Part model, mm, in its own coordinate system. A direction names the side the tool comes from. Round coordinates to 2 decimals unless told otherwise and drop trailing zeros. Loops run counter-clockwise (first coordinate to the right, second up) from the corner with the lowest first, then second, coordinate; pieces in that order, holes last. Notation, with made-up numbers: M 71,23.5 L 87,23.5 A20 cw 87,45.5 Z; hole C -13,70 d8. An arc over 180 degrees is marked long. Put each result on its own line as item: value. Start each with the question number.
1) Drop flat-ended pins along their axis: pin 1 Ø2 at (x, y) = (-1.5, -26.5) entering from -Z; pin 2 Ø1 at (x, y) = (2.5, -25) entering from -Z; pin 3 Ø0.7 at (x, z) = (-2.5, -2) entering from +Y; pin 4 Ø1.5 at (x, z) = (-1.5, -1) entering from -Y. Give the stop position or say it passes through.
2) Pull direction X, two halves, no side cores. Call faces 1 (the flat face through (-3, -36.5, -3)), 2 (the flat face through (2.8, 0, 1.9)): +X half, -X half, draft (parallel to the pull), parting line (faces both ways), or undercut.
3) Slice it at B-B on z = 0. Give the cut face in (x, y), then the cut area to 3 significant figures.
4) Which spindle directions (+Z, -Z, +X, -X, +Y, -Y) get a long thin tool onto all of the face, cutting with end or side? Do faces 3 (the flat face through (-2.7, -13.9, -2.15)), 4 (the flat face through (3.75, -14, 0)), 5 (the cylindrical face through (-3.8, -29.16, 2.11)), 6 (the flat face through (2.8, -27.5, 1.9)). Say none if no direction does.
5) Slice it at A-A on x = 0. Give the cut face in (y, z), then the cut area to 3 significant figures.
6) Probe line 1 along X through (y, z) = (0.5, 0.25); line 2 along Z through (x, y) = (0, -29.75); line 3 along Z through (x, y) = (2.75, -3.5). List the from-to ranges inside material, lowest first.
7) Slice it at C-C on y = -34.75. Give the cut face in (x, z), then the cut area to 3 significant figures.
```python
from build123d import *

# Parameters (mm, degrees)
F3_R      = 4.5
F4_DEPTH  = 27.5
F8_DEPTH  = 27.5
F6_R      = 4.5
F6_R_2    = 4
F9_DEPTH  = 9
F7_R      = 4.5
F7_R_2    = 4
F10_DEPTH = 11
F11_R     = 2.5
F11_R_2   = 0.75
F12_DEPTH = 4.501


# Not quite as in the source:
# - ends of sketch curves that miss each other by under 0.0002 mm in the source are joined


with BuildPart() as f4:
    # F3 (on Front) → F4 (new body)
    with BuildSketch(Plane.XZ):
        Circle(F3_R)
    extrude(amount=F4_DEPTH)

    # F5 (on face) → F8 (cut, through all)
    with BuildSketch(Plane.XZ.offset(27.5)):
        with BuildLine():
            Line((-1.25, -3.8), (0, -3.8))
            Line((0, -3.8), (1.25, -3.8))
            Line((1.25, -3.8), (1.25, -3.7))
            ThreePointArc((1.25, -3.7), (1.3085786438, -3.5585786438), (1.45, -3.5))
            Line((1.45, -3.5), (2, -3.5))
            Line((2, -3.5), (2, -3.05))
            ThreePointArc((2, -3.05), (2.0585786438, -2.9085786438), (2.2, -2.85))
            Line((2.2, -2.85), (3.15, -2.85))
            Line((3.15, -2.85), (3.15, -2.15))
            Line((3.15, -2.15), (2.2, -2.15))
            ThreePointArc((2.2, -2.15), (2.0585786438, -2.0914213562), (2, -1.95))
            Line((2, -1.95), (2, -1.887459))
            ThreePointArc((2, -1.887459), (2.1033535752, -1.771554046), (2.2, -1.65))
            Line((2.2, -1.65), (3.75, -1.65))
            Line((3.75, -1.65), (3.75, 0))
            Line((3.75, 0), (3.75, 1.65))
            Line((3.75, 1.65), (2.2, 1.65))
            ThreePointArc((2.2, 1.65), (2.1033535752, 1.771554046), (1.9999998047, 1.8874588157))
            Line((1.9999998047, 1.8874588157), (2, 1.95))
            ThreePointArc((2, 1.95), (2.0585786438, 2.0914213562), (2.2, 2.15))
            Line((2.2, 2.15), (3.15, 2.15))
            Line((3.15, 2.15), (3.15, 2.85))
            Line((3.15, 2.85), (2.2, 2.85))
            ThreePointArc((2.2, 2.85), (2.0585786438, 2.9085786438), (2, 3.05))
            Line((2, 3.05), (2, 3.5))
            Line((2, 3.5), (1.45, 3.5))
            ThreePointArc((1.45, 3.5), (1.3085786438, 3.5585786438), (1.25, 3.7))
            Line((1.25, 3.7), (1.25, 3.8))
            Line((1.25, 3.8), (0, 3.8))
            Line((0, 3.8), (-1.25, 3.8))
            Line((-1.25, 3.8), (-1.25, 3.7))
            ThreePointArc((-1.25, 3.7), (-1.3085786438, 3.5585786438), (-1.45, 3.5))
            Line((-1.45, 3.5), (-2, 3.5))
            Line((-2, 3.5), (-2, 3.05))
            ThreePointArc((-2, 3.05), (-2.0585786438, 2.9085786438), (-2.2, 2.85))
            Line((-2.2, 2.85), (-3.15, 2.85))
            Line((-3.15, 2.85), (-3.15, 2.15))
            Line((-3.15, 2.15), (-2.2, 2.15))
            ThreePointArc((-2.2, 2.15), (-2.0585786438, 2.0914213562), (-2, 1.95))
            Line((-2, 1.95), (-2, 1.887459))
            ThreePointArc((-2, 1.887459), (-2.1033535752, 1.771554046), (-2.2, 1.65))
            Line((-2.2, 1.65), (-3.75, 1.65))
            Line((-3.75, 1.65), (-3.75, 0))
            Line((-3.75, 0), (-3.75, -1.65))
            Line((-3.75, -1.65), (-2.2, -1.65))
            ThreePointArc((-2.2, -1.65), (-2.1033535752, -1.771554046), (-1.9999998047, -1.8874588157))
            Line((-1.9999998047, -1.8874588157), (-2, -1.95))
            ThreePointArc((-2, -1.95), (-2.0585786438, -2.0914213562), (-2.2, -2.15))
            Line((-2.2, -2.15), (-3.15, -2.15))
            Line((-3.15, -2.15), (-3.15, -2.85))
            Line((-3.15, -2.85), (-2.2, -2.85))
            ThreePointArc((-2.2, -2.85), (-2.0585786438, -2.9085786438), (-2, -3.05))
            Line((-2, -3.05), (-2, -3.5))
            Line((-2, -3.5), (-1.45, -3.5))
            ThreePointArc((-1.45, -3.5), (-1.3085786438, -3.5585786438), (-1.25, -3.7))
            Line((-1.25, -3.7), (-1.25, -3.8))
        make_face()
    extrude(amount=-F8_DEPTH, mode=Mode.SUBTRACT)

    # F6 (on face) → F9 (join)
    with BuildSketch(Plane.XZ.offset(27.5)):
        Circle(F6_R)
        Circle(F6_R_2, mode=Mode.SUBTRACT)
    extrude(amount=F9_DEPTH)

    # F7 (on face) → F10 (join)
    with BuildSketch(Plane(origin=(0, 0, 0), x_dir=(-1, 0, 0), z_dir=(0, 1, 0))):
        Circle(F7_R)
        Circle(F7_R_2, mode=Mode.SUBTRACT)
    extrude(amount=F10_DEPTH)

    # F11 (on Right) → F12 (cut, through all)
    with BuildSketch(Plane.YZ):
        with Locations((-30.5, 0)):
            Circle(F11_R)
        with Locations((-34.75, 0)):
            Circle(F11_R_2)
    extrude(amount=-F12_DEPTH, mode=Mode.SUBTRACT)


solid = f4.part
```
Recorded:
1. pin 1: stops at z = -4.47
1. pin 2: stops at z = -4.03
1. pin 3: stops at y = 0
1. pin 4: passes through
2. face 1: draft
2. face 2: undercut
3. outline: M -4.5,-36.5 L -4,-36.5 L -4,-35.5 L -4.5,-35.5 Z; M -4.5,-34 L -4,-34 L -4,-33 L -4.5,-33 Z; M -4.5,-28 L -4,-28 L -4,-27.5 L -3.75,-27.5 L -3.75,0 L -4,0 L -4,11 L -4.5,11 Z; M 3.75,-27.5 L 4,-27.5 L 4,-36.5 L 4.5,-36.5 L 4.5,11 L 4,11 L 4,0 L 3.75,0 Z
3. area: 58.0 mm2
4. face 3: +Y, -Y
4. face 4: none
4. face 5: -X
4. face 6: -Y
5. outline: M -36.5,-4.5 L 11,-4.5 L 11,-4 L 0,-4 L 0,-3.8 L -27.5,-3.8 L -27.5,-4 L -36.5,-4 Z; M -36.5,4 L -27.5,4 L -27.5,3.8 L 0,3.8 L 0,4 L 11,4 L 11,4.5 L -36.5,4.5 Z
5. area: 58.5 mm2
6. line 1: x = -4.49 to -3.99, 3.99 to 4.49
6. line 2: z = -4.5 to -4, 4 to 4.5
6. line 3: z = -3.56 to -2.85, -2.15 to -1.65, 1.65 to 2.15, 2.85 to 3.56
7. outline: M -4.44,-0.75 A4.5 ccw long -4.44,0.75 L -3.93,0.75 A4 cw long -3.93,-0.75 Z
7. area: 12.6 mm2
